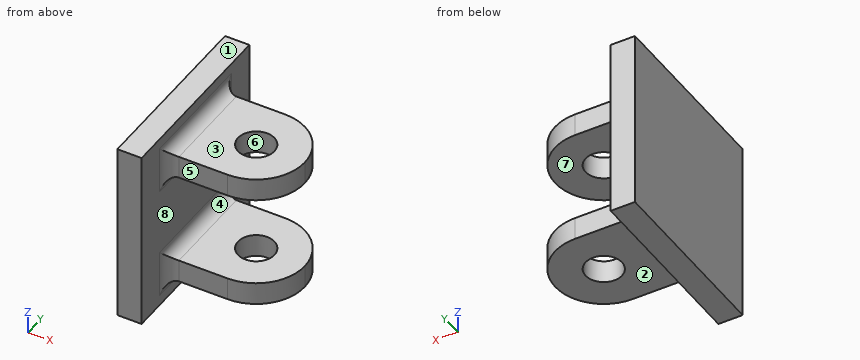
from build123d import *

# Parameters (mm, degrees)
SKETCH2_W           = 19.05
SKETCH2_H           = 19.05
BOSS_EXTRUDE2_DEPTH = 2.54
SKETCH3_W           = 2.38125
SKETCH3_H           = 10.16
BOSS_EXTRUDE3_DEPTH = 11.43
CUT_EXTRUDE1_DEPTH  = 29.912119026
SKETCH4_4_R         = 1.905
CUT_EXTRUDE2_DEPTH  = 29.912119026
FILLET3_R           = 1.27


with BuildPart() as part:
    # Sketch2 → Boss-Extrude2 (new body)
    with BuildSketch(Plane(origin=(0, 0, 0), x_dir=(0, 0, -1), z_dir=(1, 0, 0))):
        with Locations((9.525, 9.525)):
            Rectangle(SKETCH2_W, SKETCH2_H)
    extrude(amount=BOSS_EXTRUDE2_DEPTH)

    # Sketch3 → Boss-Extrude3 (add)
    with BuildSketch(Plane(origin=(2.54, 0, 0), x_dir=(0, 0, -1), z_dir=(1, 0, 0))):
        with Locations((3.571875, 9.525)):
            Rectangle(SKETCH3_W, SKETCH3_H)
        with Locations((15.478125, 9.525)):
            Rectangle(SKETCH3_W, SKETCH3_H)
    extrude(amount=BOSS_EXTRUDE3_DEPTH)

    # Sketch4 → Cut-Extrude1 (cut, through all)
    with BuildSketch(Plane.XY.offset(-2.38125)):
        with BuildLine():
            Line((13.97, 14.605), (8.89, 14.605))
            ThreePointArc((8.89, 14.605), (12.482102448, 13.117102448), (13.97, 9.525))
            Line((13.97, 9.525), (13.97, 14.605))
        make_face()
        with BuildLine():
            Line((13.97, 4.445), (13.97, 9.525))
            ThreePointArc((13.97, 9.525), (12.482102448, 5.932897552), (8.89, 4.445))
            Line((8.89, 4.445), (13.97, 4.445))
        make_face()
    extrude(amount=-CUT_EXTRUDE1_DEPTH, mode=Mode.SUBTRACT)

    # Sketch4<4> → Cut-Extrude2 (cut, through all)
    with BuildSketch(Plane.XY.offset(-2.38125)):
        with Locations((8.89, 9.525)):
            Circle(SKETCH4_4_R)
    extrude(amount=-CUT_EXTRUDE2_DEPTH, mode=Mode.SUBTRACT)

    # Fillet3
    fillet3_edges = [part.edges().sort_by_distance(p)[0] for p in [
        (2.54, 9.525, -2.38125),
        (2.54, 4.445, -3.571875),
        (2.54, 9.525, -4.7625),
        (2.54, 14.605, -3.571875),
        (2.54, 9.525, -14.2875),
        (2.54, 4.445, -15.478125),
        (2.54, 9.525, -16.66875),
        (2.54, 14.605, -15.478125),
    ]]
    fillet(fillet3_edges, radius=FILLET3_R)


solid = part.part
The model under review builds one solid part; all positions refer to its coordinate system, in mm. Face numbers are marked on the shaded views. A direction names the side the tool comes from. Round coordinates to 2 decimals unless told otherwise and drop trailing zeros. Loops run counter-clockwise (first coordinate to the right, second up) from the corner with the lowest first, then second, coordinate; pieces in that order, holes last. Notation, with made-up numbers: (62, -2) -> (89, -2) arc R23 ccw to (89, 15) -> close; hole circle Ø9 at (19.5, 29). An arc over 180 degrees is marked (long way). Write item = value, one per line. Start each with the question number.
Item 1: For the marked faces 1, 2, 3, 4 and 5, list the 3-axis set-ups (+Z, -Z, +X, -X, +Y, -Y) from which the entire face can be reached by the end or side of a thin tool; tool diameter is ignored.
Item 2: Take a section at A-A on z = -15.5. Give the boundary of the cut face in (x, y) (3 decimals).
Item 3: To check wall thickness, follow L1, parallel to Y at x = 8.89, z = -16 (3 decimals); L2, parallel to Z at x = 12, y = 10.5; L3, parallel to X at y = 6.5, z = -8.5. State the ranges of each line that lie inside material, in increasing order.
Item 4: Take a section at B-B on x = 7.25. Give the boundary of the cut face in (y, z) (1 decimal).
Item 5: Insertion check: pin 1 (3 mm diameter, centred on x = 8.89, y = 9.525, fed in from -Z); pin 2 (8 mm diameter, centred on x = 10.5, y = 9.5, fed in from +Z); pin 3 (8 mm diameter, centred on y = 5, z = -2, fed in from +X); pin 4 (9.5 mm diameter, centred on y = 5, z = -8.5, fed in from +X). Each pin has a flat end and moves straight along its axis. Give the tip position at first contact, or say it passes through.
Item 6: Mouldability with a two-part tool opening along X and no side actions: class the marked faces 6, 7 and 8 as released by +X, released by -X, zero draft, split by the parting line, or undercut.
Item 7: Take a section at C-C on y = 8.5. Give the boundary of the cut face in (x, z), plus the area to 3 significant figures.
Item 8: Take a section at D-D on x = 12.25. Give the boundary of the cut face in (y, z).
Result:
q1.face_1 = +Z, +X, -X, +Y, -Y
q1.face_2 = -Z, +X, +Y, -Y
q1.face_3 = +Z, +X, +Y, -Y
q1.face_4 = +X, +Y, -Y
q1.face_5 = +Z, -Z, +X, -Y
q2.outline = (0, 0) -> (2.54, 0) -> (2.54, 3.175) arc R1.27 cw to (3.81, 4.445) -> (8.89, 4.445) arc R5.08 ccw to (8.89, 14.605) -> (3.81, 14.605) arc R1.27 cw to (2.54, 15.875) -> (2.54, 19.05) -> (0, 19.05) -> close; hole circle Ø3.81 at (8.89, 9.525)
q3.L1 = 4.445 to 7.62, 11.43 to 14.605
q3.L2 = -16.67 to -14.29, -4.76 to -2.38
q3.L3 = 0 to 2.54
q4.outline = (4.4, -16.7) -> (8.6, -16.7) -> (8.6, -14.3) -> (4.4, -14.3) -> close; (4.4, -4.8) -> (8.6, -4.8) -> (8.6, -2.4) -> (4.4, -2.4) -> close; (10.5, -16.7) -> (14.6, -16.7) -> (14.6, -14.3) -> (10.5, -14.3) -> close; (10.5, -4.8) -> (14.6, -4.8) -> (14.6, -2.4) -> (10.5, -2.4) -> close
q5.pin_1 = through
q5.pin_2 = -2.38
q5.pin_3 = 13.94
q5.pin_4 = 13.71
q6.face_6 = undercut
q6.face_7 = zero draft
q6.face_8 = released by +X
q7.outline = (0, -19.05) -> (2.54, -19.05) -> (2.54, -17.94) arc R1.27 cw to (3.81, -16.67) -> (7.28, -16.67) -> (7.28, -14.29) -> (3.81, -14.29) arc R1.27 cw to (2.54, -13.02) -> (2.54, -6.03) arc R1.27 cw to (3.81, -4.76) -> (7.28, -4.76) -> (7.28, -2.38) -> (3.81, -2.38) arc R1.27 cw to (2.54, -1.11) -> (2.54, 0) -> (0, 0) -> close; (10.5, -16.67) -> (13.87, -16.67) -> (13.87, -14.29) -> (10.5, -14.29) -> close; (10.5, -4.76) -> (13.87, -4.76) -> (13.87, -2.38) -> (10.5, -2.38) -> close
q7.area = 88.4 mm²
q8.outline = (5.71, -16.67) -> (13.34, -16.67) -> (13.34, -14.29) -> (5.71, -14.29) -> close; (5.71, -4.76) -> (13.34, -4.76) -> (13.34, -2.38) -> (5.71, -2.38) -> close
